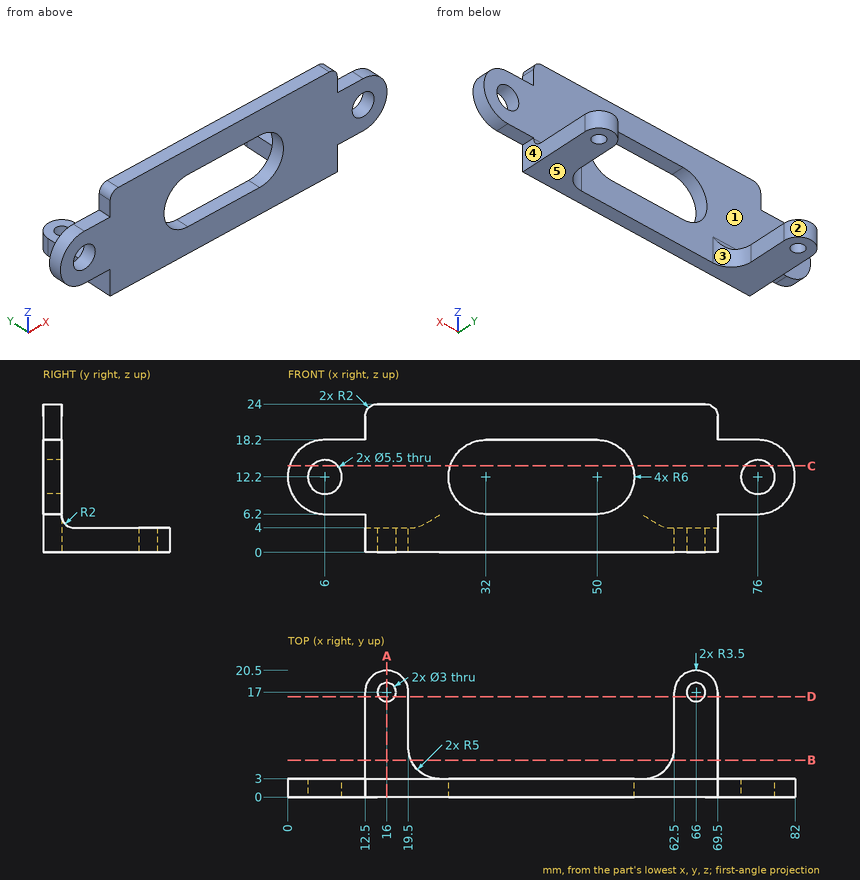
Geometry check sheet. Reference: drawing and pictorial views, mm from the part's lowest x, y, z. A direction names the side the tool comes from. Coordinates: 2 decimals unless noted, no trailing zeros. Loops run counter-clockwise (first coordinate to the right, second up) from the corner with the lowest first, then second, coordinate; pieces in that order, holes last. Notation, with made-up numbers: M 85.5,-28 L 119.5,-28 A14 ccw 119.5,-22 Z; hole C 11,61 d10. An arc over 180 degrees is marked long. One line per item, written item: value.
1. Set-up check for the marked faces 1 and 2: record each of +Z, -Z, +X, -X, +Y, -Y from which the full face is reachable in a straight line by a thin tool's end or side.
Answers follow:
face 1: +Z, +Y
face 2: +Z, -Z, +Y
2. Section check D-D on y = 16.25. Record the cut outline in (x, z), plus the area to 3 significant figures.
Answers follow:
outline: M 12.5,0 L 14.7,0 L 14.7,4 L 12.5,4 Z; M 17.3,0 L 19.5,0 L 19.5,4 L 17.3,4 Z; M 62.5,0 L 64.7,0 L 64.7,4 L 62.5,4 Z; M 67.3,0 L 69.5,0 L 69.5,4 L 67.3,4 Z
area: 35.2 mm^2
3. Section check A-A on x = 16. Record the cut outline in (y, z).
Answers follow:
outline: M 0,0 L 15.5,0 L 15.5,4 L 5,4 A2 cw 3,6 L 3,24 L 0,24 Z; M 18.5,0 L 20.5,0 L 20.5,4 L 18.5,4 Z
4. Section check C-C on z = 14. Record the cut outline in (x, y), plus the area to 3 significant figures.
Answers follow:
outline: M 0.28,0 L 3.92,0 L 3.92,3 L 0.28,3 Z; M 8.08,0 L 26.28,0 L 26.28,3 L 8.08,3 Z; M 55.72,0 L 73.92,0 L 73.92,3 L 55.72,3 Z; M 78.08,0 L 81.72,0 L 81.72,3 L 78.08,3 Z
area: 131 mm^2
5. Material ranges on line 1 along Z through (x, y) = (6, 0.8); line 2 along Y through (x, z) = (16, 0.8); line 3 along X through (y, z) = (2, 13.25), recorded low to high. Write a range as from..to.
Answers follow:
line 1: 6.2..9.45, 14.95..18.2
line 2: 0..15.5, 18.5..20.5
line 3: 0.09..3.46, 8.54..26.09, 55.91..73.46, 78.54..81.91
6. Section check B-B on y = 6. Record the cut outline in (x, z).
Answers follow:
outline: M 12.5,0 L 19.92,0 L 19.92,4 L 12.5,4 Z; M 62.08,0 L 69.5,0 L 69.5,4 L 62.08,4 Z
7. Mould release check, pull along X, two halves, no side actions. Record for the marked faces 3, 4 and 5: pulls with the +X half, pulls with the -X half, needs draft (parallel to the pull), parting line crosses it, or undercut.
Answers follow:
face 3: undercut
face 4: pulls with the +X half
face 5: needs draft
8. Gauge pin test, flat ends, axial feed: P1, Ø12, axis at x = 35.5, y = 6, coming from the -Z side; P2, Ø6, axis at y = 16, z = 7.5, coming from the +X side; P3, Ø4, axis at x = 62.5, y = 18, coming from the +Z side; P4, Ø1.2, axis at y = 13.5, z = 1, coming from the -X side. Record the tip position at first contact, or that the pin passes through.
Answers follow:
P1: z = 0
P2: through
P3: z = 4
P4: x = 12.5
